from build123d import *

# Parameters (mm, degrees)
F0_R     = 29.3168750736
F1_DEPTH = 68.326
F2_DEPTH = 203.2
F3_SIZE  = 28.956


with BuildPart() as f1:
    # F0 (on Top) → F1 (new body)
    with BuildSketch(Plane.XY):
        Circle(F0_R)
    extrude(amount=F1_DEPTH)

    # F2 (add): a face of the model
    f2_faces = [f1.faces().sort_by_distance(p)[0] for p in [
        (0, 0, 68.326),
    ]]
    extrude(f2_faces, amount=F2_DEPTH)

    # F3
    f3_edges = [f1.edges().sort_by_distance(p)[0] for p in [
        (-29.316875, 0, 271.526),
    ]]
    chamfer(f3_edges, length=F3_SIZE)


solid = f1.part
For this review, take the finished solid that the model builds, in its own axes (mm). Coordinates: 2 decimals unless noted, no trailing zeros. Order: outer loops, then holes, each group sorted by start corner. A loop starts at its lowest first (then second) coordinate and runs counter-clockwise, first axis right, second up. Notation, with made-up numbers: (55, 31) - (107, 31) arc R13 ccw to (107, 38) - close; hole circle Ø1 at (48, 63). An arc over 180 degrees is marked (long way). Use one line per item in the form item = value.
Q1. Consider section A-A (z = 71). Give the boundary of the cut face in (x, y).
Checked values:
outline = circle Ø58.63 at (0, 0)
Q2. For P1, Ø6, axis at y = -10, z = 88.5, coming from the -X side; P2, Ø10, axis at y = 5.5, z = 172, coming from the -X side; P3, Ø2, axis at x = -5.5, y = -3.5, coming from the +Z side, all flat-tipped, find the tip position at first contact; note any pin that passes through.
Checked values:
P1 = -28.47
P2 = -29.31
P3 = 266.37
Q3. For probe 1 along Y at (x, z) = (0.5, 98); probe 2 along X at (y, z) = (-11, 37); probe 3 along X at (y, z) = (3.5, 104), list the stretches that pass through material, from the lowest coordinate up. Write a range as from..to.
Checked values:
probe_1 = -29.31..29.31
probe_2 = -27.17..27.17
probe_3 = -29.11..29.11
Q4. Consider section B-B (z = 247). Give the boundary of the cut face in (x, y), then the cut area to 3 significant figures.
Checked values:
outline = circle Ø49.77 at (0, 0)
area = 1,950 mm2
